Autodesk Inventor part; units mm, degrees
ref_plane "Work Plane1" through (0, 6.1, 2.775) normal (0, 0, 1) x (1, 0, 0)
ref_plane "Work Plane2" through (0, 0, 2.6) normal (0, 0, 1) x (1, 0, 0)
ref_plane "YZ Plane" through (0, 0, 0) normal (1, 0, 0) x (0, 1, 0)
sketch "Sketch1" plane through (0, 0, 0) normal (0, 0, 1) x (1, 0, 0)
  line L0 (0, 0) -> (0, 20)
  line L1 (2.1, 0) -> (2.775, 0)
  line L2 (2.775, 0) -> (2.775, 12.2)
  line L3 (2.775, 12.2) -> (2.55, 12.2)
  line L4 (2.55, 12.2) -> (2.55, 20)
  line L5 (2.55, 20) -> (1.7, 20)
  line L6 (1.7, 20) -> (1.7, 17.8)
  line L7 (1.7, 17.8) -> (1.5, 17.8)
  line L8 (1.5, 17.8) -> (1.5, 14)
  line L9 (1.5, 14) -> (2.1, 14)
  line L10 (2.1, 14) -> (2.1, 0)
  dimension "d0" = 3.4
  dimension "d1" = 3
  dimension "d3" = 4.2
  dimension "d4" = 12.2
  dimension "d5" = 20
  dimension "d6" = 14
  dimension "d7" = 17.8
  dimension "d8" = 5.55
  dimension "d9" = 5.1
revolve "Revolution1" add sketch "Sketch1" angle 360 about axis through (0, 0, 0) along (0, 1, 0)
ref_plane "Work Plane1" through (0, 6.1, 2.775) normal (0, 0, 1) x (1, 0, 0)
sketch "Sketch2" plane through (0, 6.1, 2.775) normal (0, 0, 1) x (1, 0, 0)
  line L0 (-2.775, 6.1) -> (2.775, 6.1)
  line L1 (-2.775, -6.1) -> (2.775, -6.1)
  line L2 (-0.7265, 6.1) -> (0.7265, 6.1)
  line L3 (0.7265, 6.1) -> (0.7265, 3.7)
  line L4 (0.7265, 3.7) -> (-0.7265, 3.7)
  line L5 (-0.7265, 3.7) -> (-0.7265, 6.1)
  line L6 (0, -10.1) -> (0, 17.9)
  dimension "d12" = 9.8
  dimension "d13" = 1.453
ref_plane "Work Plane2" through (0, 0, 2.6) normal (0, 0, 1) x (1, 0, 0)
extrude "Extrusion1" cut sketch "Sketch2" against normal up to surface (0.175 mm away)
pattern_circular "Circular Pattern1" count 6 over 360 about axis through (0, 6.1, 0) along (0, -1, 0) of "Extrusion1"
properties part number "PP-06" material "ABS Plastic"
Geometry check sheet. Reference: the model listing, model coordinates, mm. A direction names the side the tool comes from. Give positions to 0.01 mm unless a question says otherwise; leave off trailing zeros. Order: outer loops, then holes, each group sorted by start corner. A loop starts at its lowest first (then second) coordinate and runs counter-clockwise, first axis right, second up. Notation, with made-up numbers: (58.5, 37.5) - (73.5, 37.5) arc R19 ccw to (73.5, 58.5) - close; hole circle Ø10 at (4, 56). An arc over 180 degrees is marked (long way). Write item = value, one per line. Start each with the question number.
1) Scan lines: L1, parallel to X at y = 6, z = 0 (3 decimals); L2, parallel to X at y = 15.4, z = 0; L3, parallel to Z at x = 0, y = 19.3. Record each from-to range of solid material in increasing order.
2) Access from +Z, -Z, +X, -X, +Y, -Y to the whole of each face (thin tool, end or side, straight path). Record for faces 1 (the cylindrical face through (1.18, 16.15, 2.26)), 2 (the cylindrical face through (-1.5, 15.87, 0.07)), 3 (the cylindrical face through (2.003, 6.902, 0.631)), 4 (the flat face through (-1.7, 0, -1.5)), 5 (the flat face through (0, 11, 2.6)).
3) Draft check along Z on faces 6 (the flat face through (2, 20, 1)), 7 (the flat face through (0, 11, -2.6)), 8 (the flat face through (1.4, 14, 0.9)). Enter one of: released by +Z, released by -Z, zero draft, split by the parting line, or undercut.
4) Section check D-D (z = 1). Enter the section's corners in (x, y), then the cut area to 3 significant figures.
5) Section check A-A (z = 0). Enter the section's corners in (x, y) (3 decimals).
6) Gauge pin test, flat ends, axial feed: pin 1 Ø1 at (x, y) = (0, 16.5) entering from +Z; pin 2 Ø1.5 at (x, y) = (1.5, 7.5) entering from -Z; pin 3 Ø0.7 at (x, y) = (0, 11.5) entering from +Z; pin 4 Ø1 at (x, z) = (0, 0) entering from +Y. Record the tip position at first contact, or that the pin passes through.
7) Section check C-C (y = 13.25). Enter the section's corners in (x, z), then the cut area to 3 significant figures.
8) Section check B-B (x = 0). Enter the section's corners in (y, z) (3 decimals).
Geometry check:
q1.L1 = -2.775 to -2.1, 2.1 to 2.775
q1.L2 = -2.55 to -1.5, 1.5 to 2.55
q1.L3 = -2.55 to -1.7, 1.7 to 2.55
q2.face_1 = +Y
q2.face_2 = +Y, -Y
q2.face_3 = -Y
q2.face_4 = +Z, -Z, +X, -X, -Y
q2.face_5 = +Z, +Y
q3.face_6 = zero draft
q3.face_7 = released by -Z
q3.face_8 = undercut
q4.outline = (-2.59, 0) - (-1.85, 0) - (-1.85, 14) - (-1.12, 14) - (-1.12, 17.8) - (-1.37, 17.8) - (-1.37, 20) - (-2.35, 20) - (-2.35, 12.2) - (-2.42, 12.2) - (-2.42, 9.8) - (-2.59, 9.8) - close; (1.12, 14) - (1.85, 14) - (1.85, 0) - (2.59, 0) - (2.59, 9.8) - (2.42, 9.8) - (2.42, 12.2) - (2.35, 12.2) - (2.35, 20) - (1.37, 20) - (1.37, 17.8) - (1.12, 17.8) - close
q4.area = 32.7 mm2
q5.outline = (-2.775, 0) - (-2.1, 0) - (-2.1, 14) - (-1.5, 14) - (-1.5, 17.8) - (-1.7, 17.8) - (-1.7, 20) - (-2.55, 20) - (-2.55, 12.2) - (-2.775, 12.2) - close; (1.5, 14) - (2.1, 14) - (2.1, 0) - (2.775, 0) - (2.775, 12.2) - (2.55, 12.2) - (2.55, 20) - (1.7, 20) - (1.7, 17.8) - (1.5, 17.8) - close
q6.pin_1 = 2.55
q6.pin_2 = -2.67
q6.pin_3 = 2.6
q6.pin_4 = through
q7.outline = circle Ø5.1 at (0, 0); hole circle Ø4.2 at (0, 0)
q7.area = 6.57 mm2
q8.outline = (0, -2.775) - (9.8, -2.775) - (9.8, -2.6) - (12.2, -2.6) - (12.2, -2.55) - (20, -2.55) - (20, -1.7) - (17.8, -1.7) - (17.8, -1.5) - (14, -1.5) - (14, -2.1) - (0, -2.1) - close; (0, 2.1) - (14, 2.1) - (14, 1.5) - (17.8, 1.5) - (17.8, 1.7) - (20, 1.7) - (20, 2.55) - (12.2, 2.55) - (12.2, 2.6) - (9.8, 2.6) - (9.8, 2.775) - (0, 2.775) - close
